Design review of the part built by this model. Coordinates are the model's own, in mm. A direction names the side the tool comes from. Coordinates: 2 decimals unless noted, no trailing zeros. Order: outer loops, then holes, each group sorted by start corner. A loop starts at its lowest first (then second) coordinate and runs counter-clockwise, first axis right, second up. Notation, with made-up numbers: (-13.75, 63.25) -> (-2.75, 63.25) arc R17 cw to (-2.75, 69.25) -> close; hole circle Ø7 at (-17, 51.5). An arc over 180 degrees is marked (long way). Use a Markdown table: item, result. Add a question column.
Q1. Add section B-B (x = -3.1). Count the separate pieces of the cut face and the enclosed holes in it, then the cut area to 3 significant figures.
Q2. The part is to be moulded in two halves that separate along X. For faces 1 (the face through (-0.5, 3, 1)), 2 (the face through (-3.5, 8.7, 4.5)), 3 (the face through (-4, 1.2, 1)), say which applies: pulls with the +X half, pulls with the -X half, needs draft (parallel to the pull), parting line crosses it, or undercut.
Q3. Wall thickness on probe 1 along Z at (x, y) = (-3.1, 0.1); probe 2 along Z at (x, y) = (-0.25, 2.75); probe 3 along Y at (x, z) = (-5, 0.75): over which ranges is each line inside the solid? List them lowest first.
Q4. Insertion check: pin 1 (1.2 mm diameter, centred on y = 2.5, z = 1.5, fed in from -X); pin 2 (1.6 mm diameter, centred on x = -3.45, z = 1.45, fed in from +Y). Each pin has a flat end and moves straight along its axis. Give the tip position at first contact, or say it passes through.
Q5. Machinability: for faces 4 (the face through (-3.5, 8.7, 3.6)), 5 (the face through (-2.3, 3, 1)), 6 (the face through (-0.5, 3, 4)), which of the approach directions +Z, -Z, +X, -X, +Y, -Y give a long, thin tool a straight path to every point of the face, cutting with its end or side? Answer none if there is none.
Q6. Add section A-A (y = 5.75). State the section outline as (x, z) points, then the cut area to 3 significant figures.
Q7. Add section C-C (x = -1). State the section outline as (y, z) points, then the cut area to 3 significant figures.
Autodesk Inventor part; units mm, degrees
ref_plane "Work Plane2" through (0, 0, 4.02) normal (0, 0, 1) x (1, 0, 0)
ref_plane "YZ Plane" through (0, 0, 0) normal (1, 0, 0) x (0, 1, 0)
ref_plane "XZ Plane" through (0, 0, 0) normal (0, 1, 0) x (-1, 0, 0)
sketch "Sketch1" plane through (0, 0, 0) normal (0, 0, 1) x (1, 0, 0)
  line L0 (0, 0) -> (0, 3.3)
  line L1 (0, 3.3) -> (-1.8, 8.8)
  line L2 (-1.8, 8.8) -> (-5.1, 8.8)
  line L3 (-5.1, 8.8) -> (-5.7, 5.3)
  line L4 (-5.7, 5.3) -> (-6.2, 5.3)
  line L5 (-6.2, 5.3) -> (-6.2, 0)
  line L6 (-6.2, 0) -> (0, 0)
  dimension "d0" = 3.3
  dimension "d1" = 3.3
  dimension "d2" = 8.8
  dimension "d3" = 1.8
  dimension "d4" = 5.3
  dimension "d5" = 6.2
  dimension "d6" = 0.5
extrude "Extrusion1" add sketch "Sketch1" along normal blind 5.5
ref_plane "Work Plane2" through (0, 0, 4.02) normal (0, 0, 1) x (1, 0, 0)
ref_plane "Work Plane1" through (0, 0, 2.75) normal (0, 0, 1) x (1, 0, 0)
sketch "Sketch3" plane through (0, 0, 4.02) normal (0, 0, 1) x (1, 0, 0)
  line L0 (-6.2, 5.3) -> (-6.2, 0)
  line L1 (-6.2, 5.1) -> (-5.2, 4.1)
  line L2 (-5.2, 4.1) -> (-2.3, 4.1)
  line L3 (-2.3, 4.1) -> (-2.3, 1.2)
  line L4 (-2.3, 1.2) -> (-5.2, 1.2)
  line L5 (-5.2, 1.2) -> (-6.2, 0.2)
  line L6 (-6.2, 5.1) -> (-6.2, 0.2)
  line L7 (-5.7, 5.3) -> (-6.2, 5.3)
  line L8 (-6.2, 0) -> (0, 0)
  line L9 (-6.2, 2.65) -> (0, 2.65) construction
  line L10 (0, 0) -> (0, 3.3) construction
  dimension "d10" = 0.2
  dimension "d11" = 0.2
  dimension "d12" = 1
  dimension "d13" = 1
extrude "Extrusion2" cut sketch "Sketch3" along normal mid plane 2.3
mirror "Mirror1" about plane through (0, 0, 2.75) normal (0, 0, 1) of "Extrusion2"
sketch "Sketch4" plane through (0, 0, 0) normal (1, 0, 0) x (0, 0, -1)
  line L0 (-4.85, 4.55) -> (-3.25, 4.55)
  line L1 (-3.25, 4.55) -> (-3.25, 2.05)
  line L2 (-3.25, 2.05) -> (-4.85, 2.05)
  line L3 (-4.85, 2.05) -> (-4.85, 4.55)
  line L4 (-4.85, 4.55) -> (-3.25, 2.05) construction
  line L5 (-3.25, 4.55) -> (-4.85, 2.05) construction
  line L6 (-2.25, 4.55) -> (-0.65, 4.55)
  line L7 (-0.65, 4.55) -> (-0.65, 2.05)
  line L8 (-0.65, 2.05) -> (-2.25, 2.05)
  line L9 (-2.25, 2.05) -> (-2.25, 4.55)
  line L10 (-2.25, 4.55) -> (-0.65, 2.05) construction
  line L11 (-0.65, 4.55) -> (-2.25, 2.05) construction
  line L12 (0, 8.8) -> (-5.5, 8.8) construction
  line L13 (-2.75, 8.8) -> (-2.75, 0) construction
  line L14 (0, 0) -> (-5.5, 0) construction
  line L15 (0, 3.3) -> (-5.5, 3.3) construction
  point P0 (-4.05, 3.3)
  point P1 (-1.45, 3.3)
  dimension "d16" = 1.6
  dimension "d17" = 2.5
  dimension "d18" = 1
extrude "Extrusion3" cut sketch "Sketch4" against normal blind 0.5
sketch "Sketch5" plane through (-5.1, 8.8, 0) normal (0, 1, 0) x (1, 0, 0)
  circle A0 centre (1.65, -4.05) radius 1
  line L0 (-1.1, -5.5) -> (5.1, -5.5) construction
  line L1 (3.3, 0) -> (3.3, -5.5) construction
  line L2 (0, -5.5) -> (3.3, -5.5) construction
  line L3 (3.3, -5.5) -> (3.3, 0) construction
  line L4 (3.3, 0) -> (0, 0) construction
  line L5 (0, 0) -> (0, -5.5) construction
  line L6 (1.65, -5.5) -> (1.65, 0) construction
  line L7 (0, 0) -> (0, -5.5) construction
  line L8 (0, -2.75) -> (3.3, -2.75) construction
  line L9 (0.655, -4.15) -> (2.645, -4.15)
  line L10 (2.645, -3.95) -> (0.655, -3.95)
  circle A1 centre (1.65, -1.45) radius 1
  line L11 (1.65, 0) -> (1.65, -5.5) construction
  line L12 (0.655, -1.35) -> (2.645, -1.35)
  line L13 (2.645, -1.55) -> (0.655, -1.55)
  point P0 (5.1, 0)
  dimension "d21" = 2
  dimension "d22" = 0.2
  dimension "d23" = 1.3
  dimension "d24" = 0.1
extrude "Extrusion4" cut sketch "Sketch5" against normal blind 0.1 contours L10 A0 | A0 L9 | L12 A1 | A1 L13
extrude "Extrusion5" cut sketch "Sketch5" against normal blind 0.2 contours A0 L9 L10 | A1 L13 L12
sketch "Sketch6" plane through (-6.2, 0, 0) normal (0, -1, 0) x (1, 0, 0)
  circle A0 centre (3.1, 4.02) radius 0.35
  circle A1 centre (3.1, 1.48) radius 0.35
  line L0 (6.2, 2.25) -> (6.2, 3.25) construction
  line L1 (6.2, 2.75) -> (0, 2.75) construction
  line L2 (0, 2.63) -> (1, 2.63) construction
  line L3 (6.2, 0) -> (6.2, 5.5) construction
  dimension "d29" = 0.7
  dimension "d30" = 2.54
  dimension "d31" = 3.1
extrude "Extrusion6" cut sketch "Sketch6" against normal blind 0.2
properties part number "CAN_bus_wire"
Established:
| question | item | result |
|---|---|---|
| 1 | separate pieces | 1 |
| 1 | enclosed holes | 2 |
| 1 | area | 34.4 mm^2 |
| 2 | face 1 | pulls with the +X half |
| 2 | face 2 | undercut |
| 2 | face 3 | needs draft |
| 3 | probe 1 | 0 to 1.13, 1.83 to 3.67, 4.37 to 5.5 |
| 3 | probe 2 | 0 to 0.65, 2.25 to 3.25, 4.85 to 5.5 |
| 3 | probe 3 | 0 to 1.2, 4.1 to 8.8 |
| 4 | pin 1 | x = -2.3 |
| 4 | pin 2 | y = 8.7 |
| 5 | face 4 | +Y |
| 5 | face 5 | -X |
| 5 | face 6 | +X |
| 6 | outline | (-5.62, 0) -> (-0.8, 0) -> (-0.8, 5.5) -> (-5.62, 5.5) -> close |
| 6 | area | 26.5 mm^2 |
| 7 | outline | (0, 0) -> (6.36, 0) -> (6.36, 5.5) -> (0, 5.5) -> close |
| 7 | area | 35.0 mm^2 |
